```python
from build123d import *

# Parameters (mm, degrees)
SKETCH1_R           = 1.5
BOSS_EXTRUDE1_DEPTH = 3
BOSS_EXTRUDE2_DEPTH = 6
SKETCH3_R           = 15.5
CUT_EXTRUDE1_DEPTH  = 7.5


with BuildPart() as part:
    # Sketch1 → Boss-Extrude1 (new body)
    with BuildSketch(Plane(origin=(0, 0, 0), x_dir=(1, 0, 0), z_dir=(0, 1, 0))):
        with BuildLine():
            Line((12.998335315, -22.998335315), (-12.001664685, -22.998335315))
            ThreePointArc((-12.001664685, -22.998335315), (-19.072732497, -20.069403127), (-22.001664685, -12.998335315))
            Line((-22.001664685, -12.998335315), (-22.001664685, 12.001664685))
            ThreePointArc((-22.001664685, 12.001664685), (-19.072732497, 19.072732497), (-12.001664685, 22.001664685))
            Line((-12.001664685, 22.001664685), (12.998335315, 22.001664685))
            ThreePointArc((12.998335315, 22.001664685), (20.069403127, 19.072732497), (22.998335315, 12.001664685))
            Line((22.998335315, 12.001664685), (22.998335315, -12.998335315))
            ThreePointArc((22.998335315, -12.998335315), (20.069403127, -20.069403127), (12.998335315, -22.998335315))
        make_face()
        with Locations(Location((-14.501664685, 14.501664685, 0), (0, 0, 270))):
            Circle(SKETCH1_R, mode=Mode.SUBTRACT)
        with Locations(Location((15.498335315, 14.501664685, 0), (0, 0, 90))):
            Circle(SKETCH1_R, mode=Mode.SUBTRACT)
        with Locations(Location((15.498335315, -15.498335315, 0), (0, 0, 270))):
            Circle(SKETCH1_R, mode=Mode.SUBTRACT)
        with Locations(Location((-14.501664685, -15.498335315, 0), (0, 0, 90))):
            Circle(SKETCH1_R, mode=Mode.SUBTRACT)
    extrude(amount=BOSS_EXTRUDE1_DEPTH)

    # Sketch2 → Boss-Extrude2 (add)
    with BuildSketch(Plane(origin=(0, 0, 0), x_dir=(1, 0, 0), z_dir=(0, 1, 0))):
        Polygon((-6, 22.001664685), (-6, 6), (-22.001664685, 6), (-22.001664685, -6.998335315), (-6.001664685, -6.998335315), (-6.001664685, -22.998335315), (6.998335315, -22.998335315), (6.998335315, -6.998335315), (22.998335315, -6.998335315), (22.998335315, 6), (6.998335315, 6), (6.998335315, 22.001664685), align=None)
    extrude(amount=-BOSS_EXTRUDE2_DEPTH)

    # Sketch3 → Cut-Extrude1 (cut, symmetric)
    with BuildSketch(Plane(origin=(0, 0, 0), x_dir=(1, 0, 0), z_dir=(0, 1, 0))):
        with Locations(Location((0.498335315, -0.498335315, 0), (0, 0, 114.787084328))):
            Circle(SKETCH3_R)
    extrude(amount=CUT_EXTRUDE1_DEPTH, both=True, mode=Mode.SUBTRACT)


solid = part.part
```
Read the model definition and answer for the solid it produces. Units are mm, in the model's axes. A direction names the side the tool comes from. Coordinates: 2 decimals unless noted, no trailing zeros. Write each loop counter-clockwise with the first axis right and the second up, starting at its lowest first coordinate (ties: lowest second). Pieces come first, ordered by that corner, then holes. Notation, with made-up numbers: (48.5, 37.25) -> (56.5, 37.25) arc R16 ccw to (56.5, 59.25) -> close; hole circle Ø4 at (-2.5, 68.5). An arc over 180 degrees is marked (long way). Write item = value, one per line.
(1) Section C-C on z = -5 is taken. Write down the section's boundary in (x, y), plus the area to 3 significant figures.
From the geometry:
outline = (-22, -6) -> (-13.99, -6) -> (-13.99, 3) -> (-22, 3) -> close; (14.99, -6) -> (23, -6) -> (23, 3) -> (14.99, 3) -> close
area = 144 mm2
(2) Given pin 1 Ø1.8 at (x, z) = (-14.5, 15.5) entering from +Y; pin 2 Ø1.8 at (y, z) = (-2.5, -17) entering from +X; pin 3 Ø3 at (x, y) = (-16.5, -3) entering from -Z; pin 4 Ø2 at (x, y) = (18.5, -2) entering from +Z, each flat-ended and moving along its own axis, determine where each tip first touches the part or whether it passes through.
From the geometry:
pin_1 = through
pin_2 = 7
pin_3 = -6
pin_4 = 7
(3) Which of the six approach directions +Z, -Z, +X, -X, +Y, -Y give full straight-line access (tool end or side, diameter ignored) to faces 4 (the face through (6.998, -3, -18)), 5 (the face through (-6, -3, -18)), 6 (the face through (-18, -3, -6)), 7 (the face through (19, -3, 6.998))?
From the geometry:
face_4 = +Z, -Z, +X, -Y
face_5 = +Z, -Z, -X, -Y
face_6 = -Z, +X, -X, -Y
face_7 = +Z, +X, -X, -Y
(4) Section A-A on x = -4.5 is taken. Write down the section's boundary in (y, z), plus the area to 3 significant figures.
From the geometry:
outline = (-6, -22) -> (3, -22) -> (3, -14.17) -> (-6, -14.17) -> close; (-6, 15.17) -> (3, 15.17) -> (3, 23) -> (-6, 23) -> close
area = 141 mm2
(5) For a pull along Z with two mould halves and no side action, classify faces 1 (the face through (-16, 0, -16)), 2 (the face through (-15.414, 1.479, -15.692)), 3 (the face through (-19.15, 1.479, -18.995)) as +Z half, -Z half, draft (parallel to the pull), parting line (faces both ways), or undercut.
From the geometry:
face_1 = draft
face_2 = undercut
face_3 = -Z half
(6) Section B-B on y = -3.75 is taken. Write down the section's boundary in (x, z), plus the area to 3 significant figures.
From the geometry:
outline = (-22, -6) -> (-13.57, -6) arc R15.5 cw to (-13.57, 7) -> (-22, 7) -> close; (-6, -22) -> (7, -22) -> (7, -13.57) arc R15.5 cw to (-6, -13.57) -> close; (-6, 14.57) arc R15.5 cw to (7, 14.57) -> (7, 23) -> (-6, 23) -> close; (14.57, -6) -> (23, -6) -> (23, 7) -> (14.57, 7) arc R15.5 cw to start
area = 388 mm2
(7) Section D-D on y = 2 is taken. Write down the section's boundary in (x, z), plus the area to 3 significant figures.
From the geometry:
outline = (-22, -12) arc R10 ccw to (-12, -22) -> (13, -22) arc R10 ccw to (23, -12) -> (23, 13) arc R10 ccw to (13, 23) -> (-12, 23) arc R10 ccw to (-22, 13) -> close; hole circle Ø3 at (-14.5, -14.5); hole circle Ø3 at (-14.5, 15.5); hole circle Ø31 at (0.5, 0.5); hole circle Ø3 at (15.5, -14.5); hole circle Ø3 at (15.5, 15.5)
area = 1,160 mm2
(8) Straight lines are drawn through the part: L1, parallel to Z at x = 16.5, y = 2.75; L2, parallel to Z at x = -20, y = -4.25. For each, find the intervals that lie inside material, in ascending order. Write a range as from..to.
From the geometry:
L1 = -21.37..-15.62, -13.39..14.38, 16.61..22.37
L2 = -6..7
